Autodesk Inventor part; units mm, degrees
ref_plane "YZ Plane" through (0, 0, 0) normal (1, 0, 0) x (0, 1, 0)
ref_plane "XZ Plane" through (0, 0, 0) normal (0, 1, 0) x (-1, 0, 0)
ref_plane "XY Plane" through (0, 0, 0) normal (0, 0, 1) x (1, 0, 0)
sketch "スケッチ1" plane through (0, 0, 0) normal (0, 0, 1) x (1, 0, 0)
  line L0 (-25.15, -23) -> (25.15, -23)
  line L1 (25.15, -23) -> (25.15, 23)
  line L2 (25.15, 23) -> (-25.15, 23)
  line L3 (-25.15, 23) -> (-25.15, -23)
  line L4 (-25.15, -23) -> (25.15, 23) construction
  line L5 (25.15, -23) -> (-25.15, 23) construction
  line L6 (-25.15, 20) -> (25.15, 20) construction
  line L7 (-25.15, -20) -> (25.15, -20) construction
  line L8 (-25.15, 20) -> (-25.15, -20) construction
  line L9 (-20.15, 20) -> (-20.15, -17.1821)
  line L10 (-20.15, -17.1821) -> (17.3109, 20)
  line L11 (17.3109, 20) -> (-20.15, 20)
  line L12 (-20.15, -20) -> (20.15, -20) construction
  line L13 (20.15, -20) -> (20.15, 20) construction
  line L14 (20.15, 20) -> (-20.15, 20) construction
  line L15 (-20.15, 20) -> (-20.15, -20) construction
  line L16 (-20.15, -20) -> (20.15, 20) construction
  line L17 (20.15, -20) -> (-20.15, 20) construction
  line L18 (20.15, 17.1821) -> (20.15, -20)
  line L19 (20.15, -20) -> (-17.3109, -20)
  line L20 (-17.3109, -20) -> (20.15, 17.1821)
  point P0 (0, 0)
  point P1 (-25.15, 0)
  point P2 (0, 0)
  dimension "d1" = 50.3
  dimension "d3" = 40
  dimension "d5" = 3
  dimension "d9" = 5
  dimension "d16" = 3
  dimension "d17" = 2
extrude "押し出し1" add sketch "スケッチ1" along normal blind 5
fillet "フィレット1" radius 3 6 edges at (-20.15, -17.1821, 2.5) (-17.3109, -20, 2.5) (-20.15, 20, 2.5) (17.3109, 20, 2.5) (20.15, 17.1821, 2.5) (20.15, -20, 2.5)
sketch "スケッチ2" plane through (25.15, -23, 0) normal (1, 0, 0) x (0, 0, -1)
  line L0 (0, 46) -> (-5, 46)
  line L1 (-5, 0) -> (-5, 46)
  point P0 (0, 23)
  point P1 (-2.5, 3)
  point P2 (-2.5, 43)
  point P3 (-2.5, 23)
  point P4 (-2.5, 46)
  point P5 (-5, 23)
  dimension "d21" = 40
  dimension "d22" = 20
hole "穴1" at (25.15, -20, 2.5) at (25.15, 20, 2.5) at (25.15, 0, 2.5) direction (-1, 0, 0) diameter 2.459 depth 3
mirror "ミラー1" about plane through (0, 0, 0) normal (1, 0, 0) of "穴1"
equation "\"d3\" = d13"
properties part number "リンク_ふともも_サブフレーム_1_1(予備案)" material "アルミニウム 2014-T4"
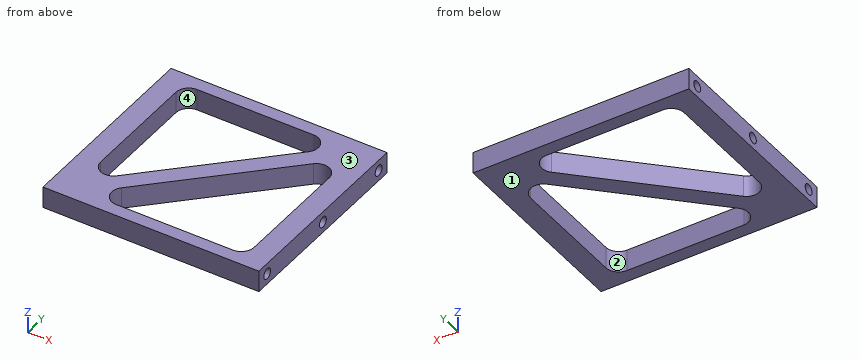
Geometry: final body of the model. Coordinates: model frame, mm. Face numbers are marked on the shaded views. A direction names the side the tool comes from. Coordinates: 2 decimals unless noted, no trailing zeros. Loops run counter-clockwise (first coordinate to the right, second up) from the corner with the lowest first, then second, coordinate; pieces in that order, holes last. Notation, with made-up numbers: M -16.75,39 L 22.25,39 A27 ccw 22.25,73 Z; hole C 47.5,43.5 d4. An arc over 180 degrees is marked long. One line per item, written item: value. Start each with the question number.
1) Reachability of the marked faces 1 and 2 from +Z, -Z, +X, -X, +Y, -Y: full face, straight path, thin tool, end or side. Return the list, or none.
2) Pin query (flat end, axial travel): P1, Ø3, axis at y = -20, z = 2.5, coming from the -X side; P2, Ø2, axis at y = 20, z = 2.5, coming from the -X side; P3, Ø0.7, axis at y = 0, z = 3, coming from the +X side. Return the tip coordinate at first contact, or that it passes through.
3) Cut plane A-A (y = 0). Return loops of the section in (x, z).
4) Cut plane B-B (z = 4.35). Return loops of the section in (x, y).
5) Cut plane D-D (x = -2). Return loops of the section in (y, z).
6) Cut plane C-C (y = -15.5). Return loops of the section in (x, z).
7) Material intervals for L1, parallel to Y at x = 24.4, z = 2.5; L2, parallel to Y at x = 7.5, z = 0.95; L3, parallel to X at y = -7.5, z = 0.2, sorted ascending. Write a range as from..to.
8) Draft query along X for the marked faces 3 and 4. Return one class per face: released by +X, released by -X, zero draft, split by the parting line, or undercut.
Evaluation:
1. face 1: -Z, +X, -X, +Y, -Y
1. face 2: +Z, -Z
2. P1: x = -25.15
2. P2: x = -22.15
2. P3: x = 22.15
3. outline: M -25.15,0 L -20.15,0 L -20.15,5 L -25.15,5 L -25.15,3.73 L -22.15,3.73 L -22.15,1.27 L -25.15,1.27 Z; M -2.84,0 L 2.84,0 L 2.84,5 L -2.84,5 Z; M 20.15,0 L 25.15,0 L 25.15,1.27 L 22.15,1.27 L 22.15,3.73 L 25.15,3.73 L 25.15,5 L 20.15,5 Z
4. outline: M -25.15,-23 L 25.15,-23 L 25.15,23 L -25.15,23 Z; hole M -20.15,-9.98 A3 ccw -15.04,-12.11 L 12.14,14.87 A3 ccw 10.03,20 L -17.15,20 A3 ccw -20.15,17 Z; hole M -12.14,-14.87 A3 ccw -10.03,-20 L 17.15,-20 A3 ccw 20.15,-17 L 20.15,9.98 A3 ccw 15.04,12.11 Z
5. outline: M -23,0 L -20,0 L -20,5 L -23,5 Z; M -4.8,0 L 0.83,0 L 0.83,5 L -4.8,5 Z; M 20,0 L 23,0 L 23,5 L 20,5 Z
6. outline: M -25.15,0 L -12.63,0 L -12.63,5 L -25.15,5 Z; M 20.15,0 L 25.15,0 L 25.15,5 L 20.15,5 Z
7. L1: -23..-21.23, -18.77..-1.23, 1.23..18.77, 21.23..23
7. L2: -23..-20, 4.63..10.26, 20..23
7. L3: -25.15..-20.15, -10.4..-4.72, 20.15..25.15
8. face 3: zero draft
8. face 4: undercut
